For this review, take the finished solid that the model builds, in its own axes (mm). Face numbers are marked on the shaded views. A direction names the side the tool comes from. Give positions to 0.01 mm unless a question says otherwise; leave off trailing zeros. Loops run counter-clockwise (first coordinate to the right, second up) from the corner with the lowest first, then second, coordinate; pieces in that order, holes last.
```python
from build123d import *

# Parameters (mm, degrees)
SKETCH2_R          = 2
CUT_EXTRUDE1_DEPTH = 5.08
CIRPATTERN1_COUNT  = 8


with BuildPart() as part:
    # Sketch1 → Revolve1 (revolve)
    with BuildSketch(Plane.XY, mode=Mode.PRIVATE) as revolve1_sk:
        Polygon((0, 8.421280131), (0, 17), (5.969, 17), (5.969, 14.8664), (9.969, 14.8664), (9.969, 17), (19.05, 17), (19.05, 14.968), (12.607925696, 3.81), (11.337925696, 3.81), (-25.706331786, 11.684), (-25.706331786, 12.954), align=None)
    revolve(revolve1_sk.sketch.rotate(Axis((0, 0, 0), (-1, 0, 0)), 90), axis=Axis((0, 0, 0), (-1, 0, 0)))

    # Sketch2 → Cut-Extrude1 (cut)
    with BuildSketch(Plane.XY.offset(17.78)):
        with Locations((13.97, 0)):
            Circle(SKETCH2_R)
    cut_extrude1 = extrude(amount=-CUT_EXTRUDE1_DEPTH, mode=Mode.SUBTRACT)

    # CirPattern1: Cut-Extrude1 ×8 about axis
    cirpattern1_axis = Axis((0, 0, 0), (1, 0, 0))
    for i in range(1, CIRPATTERN1_COUNT):
        add(cut_extrude1.rotate(cirpattern1_axis, i * 360 / CIRPATTERN1_COUNT), mode=Mode.SUBTRACT)


solid = part.part
```
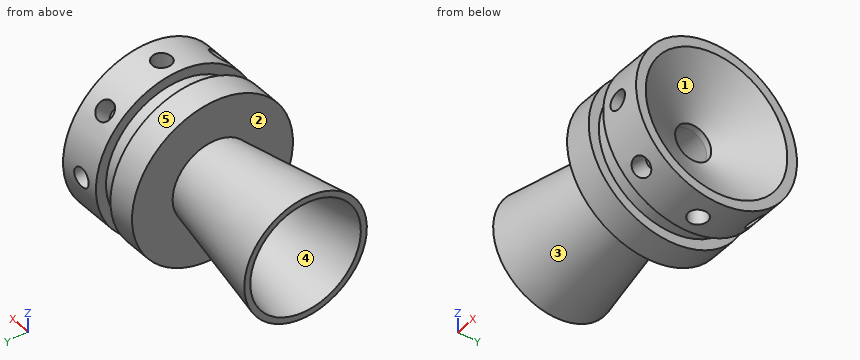
Item 1: The part is to be moulded in two halves that separate along X. For the marked faces 3, 4 and 5, say which applies: released by +X, released by -X, zero draft, split by the parting line, or undercut.
Answer:
face 3: undercut
face 4: released by -X
face 5: zero draft
Item 2: For L1, parallel to X at y = -14, z = -7.5; L2, parallel to Z at x = 13, y = -15; L3, parallel to Z at x = 2.5, y = -4.5, list the stretches that pass through material, from the lowest coordinate up.
Answer:
L1: x = 0 to 5.97, 9.97 to 19.05
L2: z = -8 to -1.75, 1.75 to 8
L3: z = -16.39 to -3.48, 3.48 to 16.39
Item 3: Tool access review of the marked faces 1 and 2: name each direction out of +Z, -Z, +X, -X, +Y, -Y from which nothing blocks a thin tool from reaching the whole face with its end or side.
Answer:
face 1: +X
face 2: none
Item 4: Clearance check with flat-ended pins moving along their axes: pin 1 Ø2 at (y, z) = (9.5, -9.5) entering from +X; pin 2 Ø2.5 at (x, y) = (13.97, 0) entering from +Z; pin 3 Ø1.2 at (x, y) = (14, -0.5) entering from -Z. State where each tip first meets the part, or that it passes through.
Answer:
pin 1: stops at x = 18.74
pin 2: stops at z = 12.7
pin 3: stops at z = -12.7
Item 5: Take a section at D-D on x = -10. Give the boundary of the cut face in (y, z).
Answer:
outline: circle Ø20.37 at (0, 0); hole circle Ø16.69 at (0, 0)
